Verification items for the finished model (mm, model axes). A direction names the side the tool comes from. Round coordinates to 2 decimals unless told otherwise and drop trailing zeros. Write each loop counter-clockwise with the first axis right and the second up, starting at its lowest first coordinate (ties: lowest second). Pieces come first, ordered by that corner, then holes. Notation, with made-up numbers: M -4,88.25 L 1,88.25 A30 ccw 1,118.25 Z; hole C 20,53.25 d7. An arc over 180 degrees is marked long. One line per item, written item: value. Start each with the question number.
Item 1: Section check A-A, the plane x = -16. Record the cut outline in (y, z).
Item 2: Section check D-D, the plane x = -5. Record the cut outline in (y, z), then the cut area to 3 significant figures.
Item 3: Section check B-B, the plane z = -13. Record the cut outline in (x, y), then the cut area to 3 significant figures.
Item 4: Section check C-C, the plane y = -132.5. Record the cut outline in (x, z), then the cut area to 3 significant figures.
Item 5: Draft check along X on faces 4 (the face through (7.15, -113.01, -10.14)), 5 (the face through (-30, -93, 11)), 6 (the face through (-20, -79, 30)). Enter one of: +X half, -X half, draft (parallel to the pull), parting line (faces both ways), or undercut.
Item 6: Gauge pin test, flat ends, axial feed: pin 1 (5 mm diameter, centred on x = -24.5, y = -89.5, fed in from -Z); pin 2 (2 mm diameter, centred on y = -105, z = 18, fed in from +X); pin 3 (10 mm diameter, centred on x = -1.5, y = -126.5, fed in from +Z). Record the tip position at first contact, or that the pin passes through.
Item 7: Thickness scan on probe 1 along Y at (x, z) = (-19.5, -18); probe 2 along Z at (x, y) = (-13, -65.5); probe 3 along X at (y, z) = (-139.5, 12). Record the ranges inside material, lowest first. Write a range as from..to.
Item 8: Tool access check on faces 1 (the face through (-20, -54, 0)), 2 (the face through (0, -130, 0)), 3 (the face through (-20, 0, 10)). Record the directions out of +Z, -Z, +X, -X, +Y, -Y that give a thin tool (end or side, any length) a straight path to the whole face; none if there is none.
from build123d import *

# Parameters (mm, degrees)
SKETCH1_W           = 20
SKETCH1_H           = 150
BOSS_EXTRUDE1_DEPTH = 30
SKETCH2_W           = 40
SKETCH2_H           = 40
BOSS_EXTRUDE2_DEPTH = 20
FILLET1_R           = 10


with BuildPart() as part:
    # Sketch1 → Boss-Extrude1 (new body)
    with BuildSketch(Plane.XY):
        with Locations((-20, -75)):
            Rectangle(SKETCH1_W, SKETCH1_H)
    extrude(amount=BOSS_EXTRUDE1_DEPTH)

    # Sketch2 → Boss-Extrude2 (add)
    with BuildSketch(Plane.XY):
        with Locations((-10, -130)):
            Rectangle(SKETCH2_W, SKETCH2_H)
    extrude(amount=-BOSS_EXTRUDE2_DEPTH)

    # Fillet1
    fillet1_edges = [part.edges().sort_by_distance(p)[0] for p in [
        (10, -110, -10),
        (-20, 0, 30),
    ]]
    fillet(fillet1_edges, radius=FILLET1_R)


solid = part.part
Response values:
1. outline: M -150,-20 L -110,-20 L -110,0 L 0,0 L 0,20 A10 ccw -10,30 L -150,30 Z
2. outline: M -150,-20 L -110,-20 L -110,0 L -150,0 Z
2. area: 800 mm2
3. outline: M -30,-150 L 10,-150 L 10,-120 A10 ccw 0,-110 L -30,-110 Z
3. area: 1,580 mm2
4. outline: M -30,-20 L 10,-20 L 10,0 L -10,0 L -10,30 L -30,30 Z
4. area: 1,400 mm2
5. face 4: +X half
5. face 5: -X half
5. face 6: draft
6. pin 1: stops at z = 0
6. pin 2: stops at x = -10
6. pin 3: stops at z = 0
7. probe 1: y = -150..-110
7. probe 2: z = 0..30
7. probe 3: x = -30..-10
8. face 1: -Z, +X, -X, +Y
8. face 2: +Z, +X, +Y, -Y
8. face 3: +Z, -Z, +X, -X, +Y
